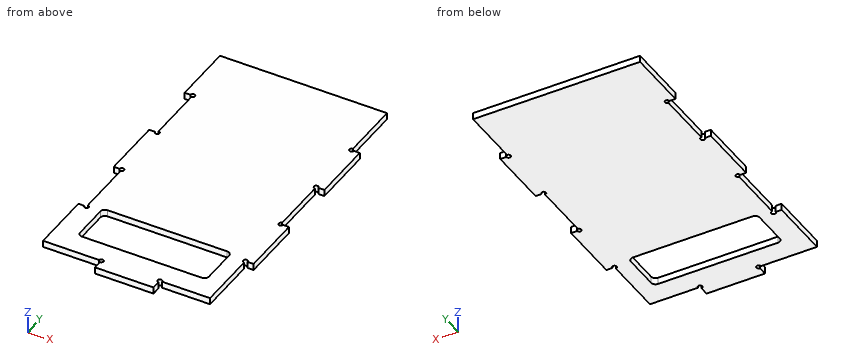
from build123d import *

# Parameters (mm, degrees)
SKETCH1_W           = 79.45
SKETCH1_H           = 140
BOSS_EXTRUDE1_DEPTH = 3
SKETCH2_W           = 58.35
SKETCH2_H           = 20
CUT_EXTRUDE1_DEPTH  = 81.542384029
FILLET1_R           = 2
SKETCH3_W           = 3.7
SKETCH3_H           = 28
CUT_EXTRUDE2_DEPTH  = 81.542384029
SKETCH5_W           = 26.5
SKETCH5_H           = 5
BOSS_EXTRUDE2_DEPTH = 3
SKETCH6_R           = 1
CUT_EXTRUDE3_DEPTH  = 85.923940235


with BuildPart() as part:
    # Sketch1 → Boss-Extrude1 (new body)
    with BuildSketch(Plane.XY):
        Rectangle(SKETCH1_W, SKETCH1_H)
    extrude(amount=BOSS_EXTRUDE1_DEPTH)

    # Sketch2 → Cut-Extrude1 (cut, through all)
    with BuildSketch(Plane.XY.offset(3)):
        with Locations((-0.55, -50)):
            Rectangle(SKETCH2_W, SKETCH2_H)
    extrude(amount=-CUT_EXTRUDE1_DEPTH, mode=Mode.SUBTRACT)

    # Fillet1
    fillet1_edges = [part.edges().sort_by_distance(p)[0] for p in [
        (28.625, -40, 1.5),
        (28.625, -60, 1.5),
        (-29.725, -60, 1.5),
        (-29.725, -40, 1.5),
    ]]
    fillet(fillet1_edges, radius=FILLET1_R)

    # Sketch3 → Cut-Extrude2 (cut, through all)
    with BuildSketch(Plane.XY.offset(3)):
        with Locations((-37.875, 28)):
            Rectangle(SKETCH3_W, SKETCH3_H)
        with Locations((-37.875, -28)):
            Rectangle(SKETCH3_W, SKETCH3_H)
        with Locations((37.875, 56)):
            Rectangle(SKETCH3_W, SKETCH3_H)
        with Locations((37.875, 0)):
            Rectangle(SKETCH3_W, SKETCH3_H)
        with Locations((37.875, -56)):
            Rectangle(SKETCH3_W, SKETCH3_H)
    extrude(amount=-CUT_EXTRUDE2_DEPTH, mode=Mode.SUBTRACT)

    # Sketch5 → Boss-Extrude2 (add)
    with BuildSketch(Plane.XY.offset(3)):
        with Locations((0, -72.5)):
            Rectangle(SKETCH5_W, SKETCH5_H)
    extrude(amount=-BOSS_EXTRUDE2_DEPTH)

    # Sketch6 → Cut-Extrude3 (cut, through all)
    with BuildSketch(Plane.XY.offset(3)):
        with Locations((-36.025, 42)):
            Circle(SKETCH6_R)
        with Locations((-36.025, 14)):
            Circle(SKETCH6_R)
        with Locations((-36.025, -14)):
            Circle(SKETCH6_R)
        with Locations((-36.025, -42)):
            Circle(SKETCH6_R)
        with Locations((-13.25, -70)):
            Circle(SKETCH6_R)
        with Locations((13.25, -70)):
            Circle(SKETCH6_R)
        with Locations((36.025, -42)):
            Circle(SKETCH6_R)
        with Locations((36.025, -14)):
            Circle(SKETCH6_R)
        with Locations((36.025, 14)):
            Circle(SKETCH6_R)
        with Locations((36.025, 42)):
            Circle(SKETCH6_R)
    extrude(amount=-CUT_EXTRUDE3_DEPTH, mode=Mode.SUBTRACT)


solid = part.part
Source: CAD feature listing. Evaluate the final solid. Frame: model axes, mm. Give positions to 0.01 mm unless a question says otherwise; leave off trailing zeros. Write each loop counter-clockwise with the first axis right and the second up, starting at its lowest first coordinate (ties: lowest second). Pieces come first, ordered by that corner, then holes. Notation, with made-up numbers: (88, -13) -> (93, -13) arc R8 cw to (93, -1) -> close; hole circle Ø9 at (85, 11.25). An arc over 180 degrees is marked (long way). Return JSON: item names as keys, results as strings. Group by question number.
1. Section B-B, the plane y = -18.5. Output: boundary loops of the cut face in (x, z) (3 decimals).
2. Pin query (flat end, axial travel): pin 1 Ø1.6 at (x, y) = (-36.025, -14) entering from +Z; pin 2 Ø0.9 at (y, z) = (-4.5, 1) entering from +X (3 decimals); pin 3 Ø0.9 at (x, z) = (-31.5, 1) entering from -Y; pin 4 Ø1.5 at (y, z) = (-74, 1) entering from -X. Return the tip coordinate at first contact, or that it passes through.
3. Material intervals for line 1 (Y direction, x = 11, z = 2.7); line 2 (Y direction, x = 16.5, z = 2.5); line 3 (X direction, y = -42.5, z = 2.55) (3 decimals), sorted ascending. Write a range as from..to.
4. Section A-A, the plane x = 18. Output: boundary loops of the cut face in (y, z).
5. Section C-C, the plane x = 8.5. Output: boundary loops of the cut face in (y, z).
Determined:
{
 "1": {"outline": "(-36.025, 0) -> (39.725, 0) -> (39.725, 3) -> (-36.025, 3) -> close"},
 "2": {"pin 1": "passes through", "pin 2": "stops at x = 36.025", "pin 3": "stops at y = -70", "pin 4": "stops at x = -13.25"},
 "3": {"line 1": "y = -75..-60, -40..70", "line 2": "y = -70..-60, -40..70", "line 3": "x = -39.725..-36.891, -35.159..-29.725, 28.625..35.159"},
 "4": {"outline": "(-70, 0) -> (-60, 0) -> (-60, 3) -> (-70, 3) -> close; (-40, 0) -> (70, 0) -> (70, 3) -> (-40, 3) -> close"},
 "5": {"outline": "(-75, 0) -> (-60, 0) -> (-60, 3) -> (-75, 3) -> close; (-40, 0) -> (70, 0) -> (70, 3) -> (-40, 3) -> close"}
}
